```python
from build123d import *

# Parameters (mm, degrees)
EXTRUDE_START       = 309
EXTRUDE_SKETCH_1_R  = 93
EXTRUDE_1_DEPTH     = 14
EXTRUDE_START_2     = 323
EXTRUDE_SKETCH_2_R  = 28
EXTRUDE_2_DEPTH     = 46
EXTRUDE_3_DEPTH     = 9
EXTRUDE_START_3     = 332
EXTRUDE_SKETCH_4_R  = 8
EXTRUDE_4_DEPTH     = 6
EXTRUDE_5_DEPTH     = 9
EXTRUDE_SKETCH_6_R  = 8
EXTRUDE_6_DEPTH     = 6
EXTRUDE_7_DEPTH     = 9
EXTRUDE_SKETCH_8_R  = 8
EXTRUDE_8_DEPTH     = 6
EXTRUDE_9_DEPTH     = 9
EXTRUDE_SKETCH_10_R = 8
EXTRUDE_10_DEPTH    = 6
EXTRUDE_SKETCH_11_R = 9
EXTRUDE_11_DEPTH    = 14
EXTRUDE_SKETCH_12_R = 9
EXTRUDE_12_DEPTH    = 14


with BuildPart() as part:
    # Extrude sketch 1 → Extrude 1 (new body)
    with BuildSketch(Plane.XY.offset(EXTRUDE_START)):
        with Locations((240, 0)):
            Circle(EXTRUDE_SKETCH_1_R)
    extrude(amount=EXTRUDE_1_DEPTH)


with BuildPart() as body_2:
    # Extrude sketch 2 → Extrude 2 (new body)
    with BuildSketch(Plane.XY.offset(EXTRUDE_START_2)):
        with Locations((240, 0)):
            Circle(EXTRUDE_SKETCH_2_R)
    extrude(amount=EXTRUDE_2_DEPTH)


with BuildPart() as body_3:
    # Revolve profile 1 → Revolve 1 (revolve)
    with BuildSketch(Plane(origin=(0, 0, 0), x_dir=(1, 0, 0), z_dir=(0, 1, 0)), mode=Mode.PRIVATE) as revolve_1_sk:
        Polygon((240, -369), (268, -369), (264, -377), (240, -380), align=None)
    revolve(revolve_1_sk.sketch.rotate(Axis((240, 0, 364), (0, 0, 1)), 180), axis=Axis((240, 0, 364), (0, 0, 1)))


with BuildPart() as body_4:
    # Extrude sketch 3 → Extrude 3 (new body)
    with BuildSketch(Plane.XY.offset(EXTRUDE_START_2)):
        Polygon((310, 30.773502692), (300, 36.547005384), (290, 30.773502692), (290, 19.226497308), (300, 13.452994616), (310, 19.226497308), align=None)
    extrude(amount=EXTRUDE_3_DEPTH)


with BuildPart() as body_5:
    # Extrude sketch 4 → Extrude 4 (new body)
    with BuildSketch(Plane.XY.offset(EXTRUDE_START_3)):
        with Locations((300, 25)):
            Circle(EXTRUDE_SKETCH_4_R)
    extrude(amount=EXTRUDE_4_DEPTH)


with BuildPart() as body_6:
    # Extrude sketch 5 → Extrude 5 (new body)
    with BuildSketch(Plane.XY.offset(EXTRUDE_START_2)):
        Polygon((310, -19.226497308), (300, -13.452994616), (290, -19.226497308), (290, -30.773502692), (300, -36.547005384), (310, -30.773502692), align=None)
    extrude(amount=EXTRUDE_5_DEPTH)


with BuildPart() as body_7:
    # Extrude sketch 6 → Extrude 6 (new body)
    with BuildSketch(Plane.XY.offset(EXTRUDE_START_3)):
        with Locations((300, -25)):
            Circle(EXTRUDE_SKETCH_6_R)
    extrude(amount=EXTRUDE_6_DEPTH)


with BuildPart() as body_8:
    # Extrude sketch 7 → Extrude 7 (new body)
    with BuildSketch(Plane.XY.offset(EXTRUDE_START_2)):
        Polygon((190, 30.773502692), (180, 36.547005384), (170, 30.773502692), (170, 19.226497308), (180, 13.452994616), (190, 19.226497308), align=None)
    extrude(amount=EXTRUDE_7_DEPTH)


with BuildPart() as body_9:
    # Extrude sketch 8 → Extrude 8 (new body)
    with BuildSketch(Plane.XY.offset(EXTRUDE_START_3)):
        with Locations((180, 25)):
            Circle(EXTRUDE_SKETCH_8_R)
    extrude(amount=EXTRUDE_8_DEPTH)


with BuildPart() as body_10:
    # Extrude sketch 9 → Extrude 9 (new body)
    with BuildSketch(Plane.XY.offset(EXTRUDE_START_2)):
        Polygon((190, -19.226497308), (180, -13.452994616), (170, -19.226497308), (170, -30.773502692), (180, -36.547005384), (190, -30.773502692), align=None)
    extrude(amount=EXTRUDE_9_DEPTH)


with BuildPart() as body_11:
    # Extrude sketch 10 → Extrude 10 (new body)
    with BuildSketch(Plane.XY.offset(EXTRUDE_START_3)):
        with Locations((180, -25)):
            Circle(EXTRUDE_SKETCH_10_R)
    extrude(amount=EXTRUDE_10_DEPTH)


with BuildPart() as body_12:
    # Extrude sketch 11 → Extrude 11 (new body)
    with BuildSketch(Plane.XY.offset(EXTRUDE_START_2)):
        with Locations((240, 75)):
            Circle(EXTRUDE_SKETCH_11_R)
    extrude(amount=EXTRUDE_11_DEPTH)


with BuildPart() as body_13:
    # Extrude sketch 12 → Extrude 12 (new body)
    with BuildSketch(Plane.XY.offset(EXTRUDE_START_2)):
        with Locations((240, -75)):
            Circle(EXTRUDE_SKETCH_12_R)
    extrude(amount=EXTRUDE_12_DEPTH)


with BuildPart() as body_10_1:
    add(body_10.part)

    # Combine _weld _ assembly of features: union body 4, body 9, body 5, body 11, body 2, body 12, body 8, body 6, body 3, body 13, body 7, part
    add(body_4.part)
    add(body_9.part)
    add(body_5.part)
    add(body_11.part)
    add(body_2.part)
    add(body_12.part)
    add(body_8.part)
    add(body_6.part)
    add(body_3.part)
    add(body_13.part)
    add(body_7.part)
    add(part.part)


solid = body_10_1.part
```
Read the model definition and answer for the solid it produces. Units are mm, in the model's axes. A direction names the side the tool comes from. Give positions to 0.01 mm unless a question says otherwise; leave off trailing zeros. Loops run counter-clockwise (first coordinate to the right, second up) from the corner with the lowest first, then second, coordinate; pieces in that order, holes last.
Item 1: The part is cut by section D-D (y = -41). Write down the section's boundary in (x, z), and give its area (3 significant figures).
Item 2: Find the intervals of material crossed by line 1 along X through (y, z) = (1.5, 365); line 2 along Z through (x, y) = (199, 82); line 3 along Y through (x, z) = (178, 331), in increasing order.
Item 3: Each of these flat-tipped pins is pushed along its axis until it touches: pin 1 Ø9 at (x, y) = (239.5, -72) entering from +Z; pin 2 Ø7 at (y, z) = (-25, 329) entering from -X; pin 3 Ø10 at (x, y) = (302, 19.5) entering from +Z. Where does it stop, or does it pass through?
Item 4: The part is cut by section C-C (x = 304.5). Write down the section's boundary in (y, z).
Item 5: For faces 4 (the flat face through (175.5, 18.2, 332)), 5 (the flat face through (304.93, 16.3, 327.44)), 6 (the flat face through (190, 25, 327)), 7 (the flat face through (184.93, -33.7, 327.44)), determine the directions among +Z, -Z, +X, -X, +Y, -Y from which every point of the face is accessible in a straight line to the end or side of a thin tool.
Item 6: The part is cut by section B-B (y = -75). Write down the section's boundary in (x, z), and give its area (3 significant figures).
Item 7: The mould has two halves that part along Y. Classify faces 1 (the flat face through (305.07, 33.62, 327.44)), 2 (the cylindrical face through (232.86, 69.52, 329.9)), 3 (the flat face through (294.93, -33.62, 327.44)): released by +Y, released by -Y, zero draft, split by the parting line, or undercut.
Item 8: The part is cut by section A-A (z = 325.5). Write down the section's boundary in (x, y).
Taken from the geometry:
1. outline: (156.53, 309) - (323.47, 309) - (323.47, 323) - (156.53, 323) - close
1. area: 2,340 mm2
2. line 1: x = 212.04 to 267.96
2. line 2: z = 309 to 323
2. line 3: y = -35.39 to -14.61, 14.61 to 35.39
3. pin 1: stops at z = 337
3. pin 2: stops at x = 170
3. pin 3: stops at z = 338
4. outline: (-67, 309) - (67, 309) - (67, 323) - (33.95, 323) - (33.95, 332) - (31.61, 332) - (31.61, 338) - (18.39, 338) - (18.39, 332) - (16.05, 332) - (16.05, 323) - (-16.05, 323) - (-16.05, 332) - (-18.39, 332) - (-18.39, 338) - (-31.61, 338) - (-31.61, 332) - (-33.95, 332) - (-33.95, 323) - (-67, 323) - close
5. face 4: +Z
5. face 5: +Z, +X
5. face 6: +Z, +Y, -Y
5. face 7: +Z, -Y
6. outline: (185.01, 309) - (294.99, 309) - (294.99, 323) - (249, 323) - (249, 337) - (231, 337) - (231, 323) - (185.01, 323) - close
6. area: 1,790 mm2
7. face 1: released by +Y
7. face 2: undercut
7. face 3: released by -Y
8. outline: (170, -30.77) - (180, -36.55) - (190, -30.77) - (190, -19.23) - (180, -13.45) - (170, -19.23) - close; (170, 19.23) - (180, 13.45) - (190, 19.23) - (190, 30.77) - (180, 36.55) - (170, 30.77) - close; circle Ø56 at (240, 0); circle Ø18 at (240, -75); circle Ø18 at (240, 75); (290, -30.77) - (300, -36.55) - (310, -30.77) - (310, -19.23) - (300, -13.45) - (290, -19.23) - close; (290, 19.23) - (300, 13.45) - (310, 19.23) - (310, 30.77) - (300, 36.55) - (290, 30.77) - close
